from build123d import *

# Parameters (mm, degrees)
F1_DEPTH = 4.7625


with BuildPart() as f1:
    # F0 (on Top) → F1 (new body, symmetric)
    with BuildSketch(Plane.XY):
        with BuildLine():
            Line((26.7500709742, -3.175), (37.6112871062, -3.175))
            Line((37.6112871062, -3.175), (41.275, 0.3440350712))
            Line((41.275, 0.3440350712), (41.275, 3.175))
            Line((41.275, 3.175), (-41.275, 3.175))
            Line((-41.275, 3.175), (-41.275, 0))
            Line((-41.275, 0), (-3.3075221407, -3.175))
            ThreePointArc((-3.3075221407, -3.175), (0.0796335022, -1.82683754), (3.466789145, -3.175))
            Line((3.466789145, -3.175), (15.9728042781, -3.175))
            ThreePointArc((15.9728042781, -3.175), (21.3614376262, -1.2663040308), (26.7500709742, -3.175))
        make_face()
    extrude(amount=F1_DEPTH, both=True)


solid = f1.part
Here's how the part is built. I have some questions about the finished solid (model axes, mm). Round coordinates to 2 decimals unless told otherwise and drop trailing zeros. Order: outer loops, then holes, each group sorted by start corner. A loop starts at its lowest first (then second) coordinate and runs counter-clockwise, first axis right, second up. Notation, with made-up numbers: M -30.75,51 L -16.75,51 A20 cw -16.75,60 Z; hole C 10.25,-32.75 d1. An arc over 180 degrees is marked long. One line per question, with ' | ' between items.
1) Imagine slicing it at B-B, the plane x = -1.5. Write out the boundary of the cut face in (y, z) (1 decimal), plus the area to 3 significant figures.
Checked values:
outline: M -2.1,-4.8 L 3.2,-4.8 L 3.2,4.8 L -2.1,4.8 Z | area: 50.1 mm²
2) Imagine slicing it at A-A, the plane z = -4. Write out the boundary of the cut face in (x, y) (3 decimals), plus the area to 3 significant figures.
Checked values:
outline: M -41.275,0 L -3.308,-3.175 A4.929 cw 3.467,-3.175 L 15.973,-3.175 A8.561 cw 26.75,-3.175 L 37.611,-3.175 L 41.275,0.344 L 41.275,3.175 L -41.275,3.175 Z | area: 437 mm²
3) Imagine slicing it at C-C, the plane x = -15. Write out the boundary of the cut face in (y, z) (1 decimal), plus the area to 3 significant figures.
Checked values:
outline: M -2.2,-4.8 L 3.2,-4.8 L 3.2,4.8 L -2.2,4.8 Z | area: 51.2 mm²
4) We'd pull the mould along X, two halves only. Please class faces 1 (the flat face through (-1, 1, 4.762)), 2 (the cylindrical face through (21.28, -1.267, 0.067)), 3 (the flat face through (-41.275, 2, 0)): released by +X, released by -X, zero draft, split by the parting line, or undercut.
Checked values:
face 1: zero draft | face 2: undercut | face 3: released by -X
5) I need wall thicknesses on line 1 (Y direction, x = -26, z = 2) (3 decimals); line 2 (Y direction, x = -29.5, z = -2.75) (3 decimals). Which ranges of each line are inside material? Lowest first, please.
Checked values:
line 1: y = -1.277 to 3.175 | line 2: y = -0.985 to 3.175
